The figure shows three views and two pictorial views of one solid part (mm, origin at its lowest corner). Answer the questions. Round coordinates to 2 decimals unless told otherwise and drop trailing zeros. Order: outer loops, then holes, each group sorted by start corner. A loop starts at its lowest first (then second) coordinate and runs counter-clockwise, first axis right, second up. Notation, with made-up numbers: (77, 84) -> (101, 84) arc R21 ccw to (101, 91) -> close; hole circle Ø2 at (34.25, 18). An arc over 180 degrees is marked (long way). One line per item, written item: value. Start each with the question number.
1. Section A-A (x = 35) is taken. Give the vertices of the cut face in (y, z), then the cut area to 3 significant figures.
2. Section B-B (y = 62) is taken. Give the vertices of the cut face in (x, z).
3. The mould has two halves that part along X. Classify the marked faces 1, 2 and 3: released by +X, released by -X, zero draft, split by the parting line, or undercut.
4. Consider line 1 (X direction, y = 65, z = 53) (1 decimal); line 2 (X direction, y = 70, z = 56) (1 decimal). Determine where each line is inside the solid, lowest interval first.
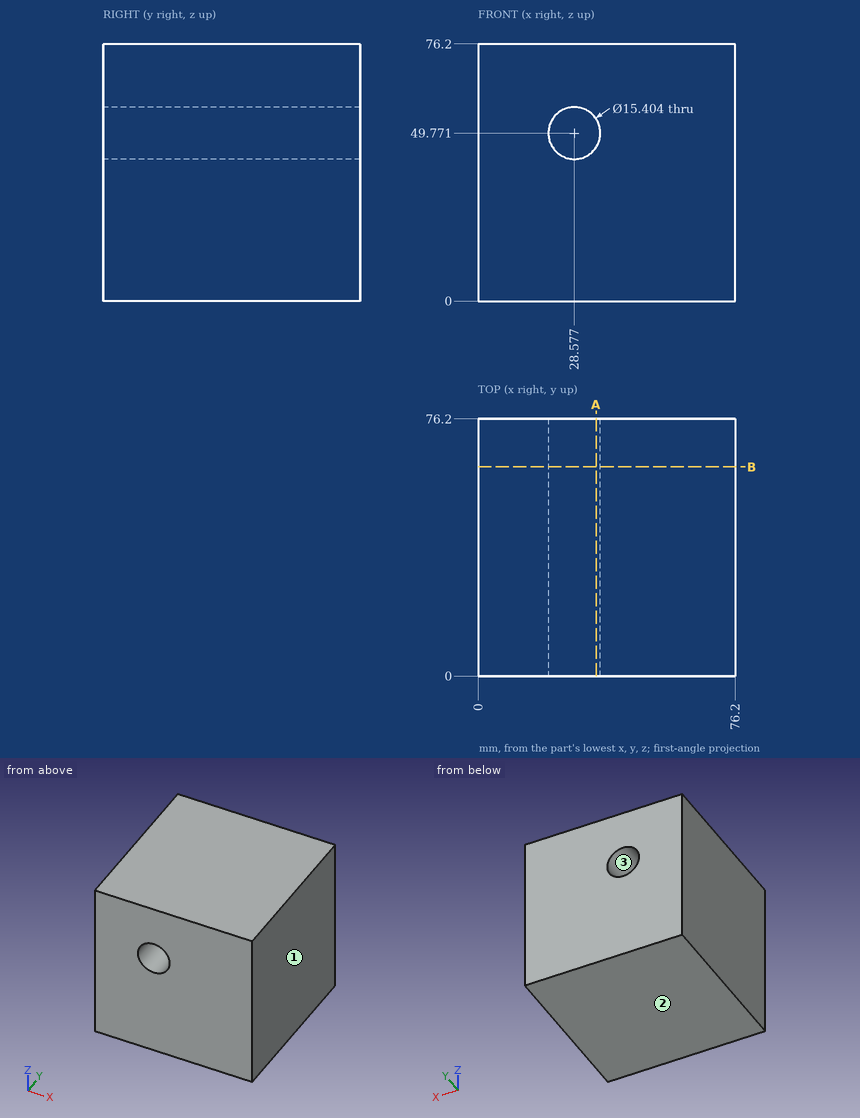
Answer:
1. outline: (0, 0) -> (76.2, 0) -> (76.2, 45.52) -> (0, 45.52) -> close; (0, 54.02) -> (76.2, 54.02) -> (76.2, 76.2) -> (0, 76.2) -> close
1. area: 5,160 mm^2
2. outline: (0, 0) -> (76.2, 0) -> (76.2, 76.2) -> (0, 76.2) -> close; hole circle Ø15.4 at (28.58, 49.77)
3. face 1: released by +X
3. face 2: zero draft
3. face 3: undercut
4. line 1: 0 to 21.6, 35.6 to 76.2
4. line 2: 0 to 24, 33.1 to 76.2
